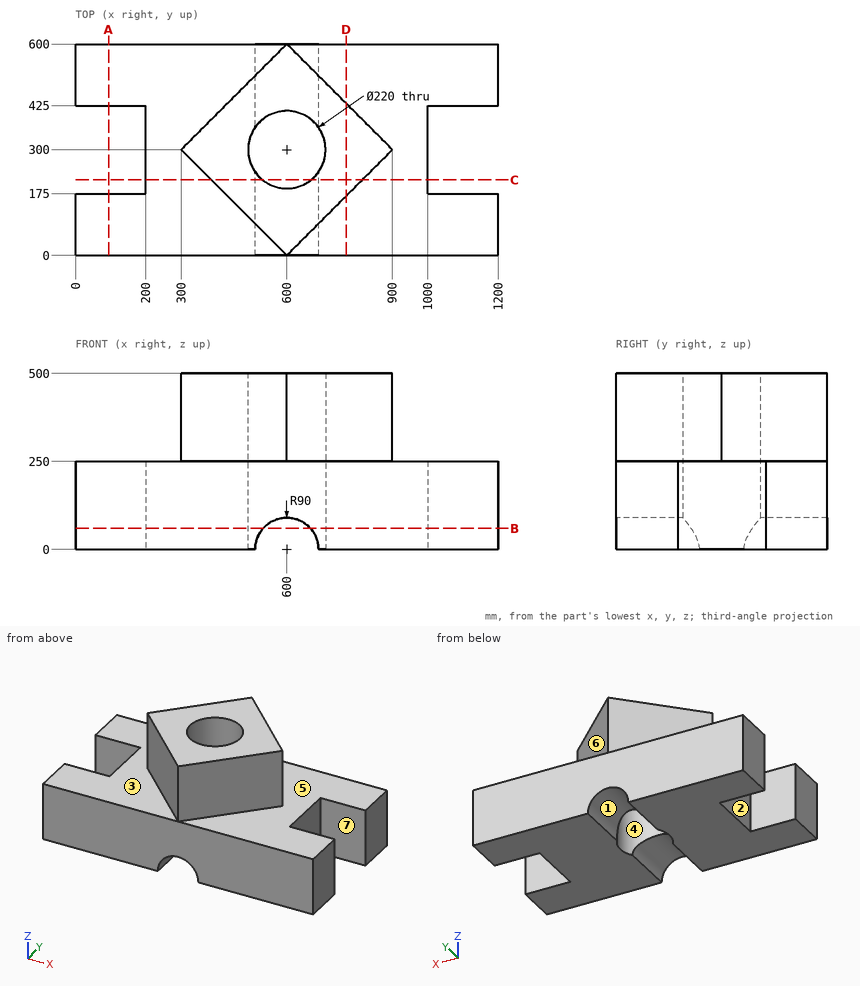
Drawing for the job (mm, zero at the part's lowest x, y, z). A direction names the side the tool comes from. Coordinates: 2 decimals unless noted, no trailing zeros. Write each loop counter-clockwise with the first axis right and the second up, starting at its lowest first coordinate (ties: lowest second). Pieces come first, ordered by that corner, then holes. Notation, with made-up numbers: (48, -24.75) - (65, -24.75) arc R27 ccw to (65, -8.75) - close; hole circle Ø9 at (28, 35). An arc over 180 degrees is marked (long way). Write each question's results on one line, items separated by ' | '. Start each with the question number.
1) Flat gauge pins, fed straight in: P1, Ø12, axis at x = 628, z = 357, coming from the -Y side; P2, Ø12, axis at y = 322, z = 87.5, coming from the +X side; P3, Ø1, axis at x = 522.5, z = 352.5, coming from the -Y side. Where does each tip first touch, or does it go through?
2) Probe line 1 along Y through (x, z) = (600, 259); line 2 along Y through (x, z) = (96, 219.5); line 3 along Z through (x, y) = (330, 419). List the from-to ranges inside material, lowest first. Write a range as from..to.
3) Cut at C-C (y = 214). Write the cut outline in (x, z), then the cut area to 3 significant figures.
4) 3-axis set-ups, long thin cutter, end or side, ignore diameter. For the marked faces 5, 6 and 7: which of +Z, -Z, +X, -X, +Y, -Y reach the whole face in a straight line?
5) Cut at D-D (x = 768). Write the cut outline in (y, z).
6) Cut at A-A (x = 94). Write the cut outline in (y, z), then the cut area to 3 significant figures.
7) Mould opens along X. For the marked faces 1, 2, 3 and 4 say: pulls with the +X half, pulls with the -X half, needs draft (parallel to the pull), parting line crosses it, or undercut.
8) Cut at B-B (z = 60). Write the cut outline in (x, y).
Returned:
1) P1: y = 22 | P2: x = 1000 | P3: y = 77
2) line 1: 0..190, 410..600 | line 2: 0..175, 425..600 | line 3: 0..250
3) outline: (200, 0) - (510, 0) arc R90 cw to (531.41, 58.28) - (531.41, 500) - (386, 500) - (386, 250) - (200, 250) - close; (668.59, 58.28) arc R90 cw to (690, 0) - (1000, 0) - (1000, 250) - (814, 250) - (814, 500) - (668.59, 500) - close | area: 237,000 mm^2
4) face 5: +Z, +X | face 6: +Z, +X, +Y | face 7: +Z, -Z, +X
5) outline: (0, 0) - (600, 0) - (600, 250) - (432, 250) - (432, 500) - (168, 500) - (168, 250) - (0, 250) - close
6) outline: (0, 0) - (175, 0) - (175, 250) - (0, 250) - close; (425, 0) - (600, 0) - (600, 250) - (425, 250) - close | area: 87,500 mm^2
7) face 1: undercut | face 2: pulls with the -X half | face 3: needs draft | face 4: undercut
8) outline: (0, 0) - (532.92, 0) - (532.92, 212.82) arc R110 cw to (532.92, 387.18) - (532.92, 600) - (0, 600) - (0, 425) - (200, 425) - (200, 175) - (0, 175) - close; (667.08, 0) - (1200, 0) - (1200, 175) - (1000, 175) - (1000, 425) - (1200, 425) - (1200, 600) - (667.08, 600) - (667.08, 387.18) arc R110 cw to (667.08, 212.82) - close
